For this review, take the finished solid that the model builds, in its own axes (mm). Face numbers are marked on the shaded views. A direction names the side the tool comes from. Give positions to 0.01 mm unless a question says otherwise; leave off trailing zeros. Loops run counter-clockwise (first coordinate to the right, second up) from the corner with the lowest first, then second, coordinate; pieces in that order, holes last.
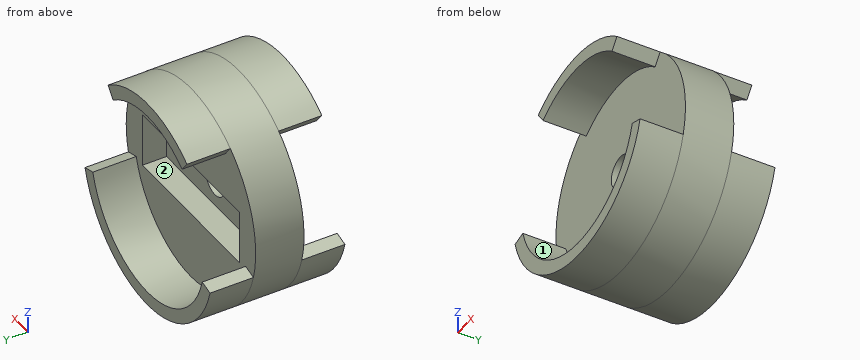
```python
from build123d import *

# Parameters (mm, degrees)
SKETCH1_R           = 25.4
SKETCH1_W           = 38.0365
SKETCH1_H           = 12.7508
BOSS_EXTRUDE1_DEPTH = 5.6642
SKETCH1_3_R         = 25.4
SKETCH1_3_W         = 38.0365
SKETCH1_3_H         = 12.7508
SKETCH1_3_R_2       = 3.71475
BOSS_EXTRUDE2_DEPTH = 5.715
BOSS_EXTRUDE3_DEPTH = 15.875


with BuildPart() as part:
    # Sketch1 → Boss-Extrude1 (new body)
    with BuildSketch(Plane(origin=(0, 0, 0), x_dir=(1, 0, 0), z_dir=(0, 1, 0))):
        Circle(SKETCH1_R)
        Rectangle(SKETCH1_W, SKETCH1_H, mode=Mode.SUBTRACT)
    extrude(amount=BOSS_EXTRUDE1_DEPTH)

    # Sketch1_3 → Boss-Extrude2 (add)
    with BuildSketch(Plane(origin=(0, 0, 0), x_dir=(1, 0, 0), z_dir=(0, 1, 0))):
        Circle(SKETCH1_3_R)
        Rectangle(SKETCH1_3_W, SKETCH1_3_H, mode=Mode.SUBTRACT)
        Rectangle(SKETCH1_3_W, SKETCH1_3_H)
        Circle(SKETCH1_3_R_2, mode=Mode.SUBTRACT)
    extrude(amount=-BOSS_EXTRUDE2_DEPTH)

    # Sketch2 → Boss-Extrude3 (add, symmetric)
    with BuildSketch(Plane(origin=(0, 0, 0), x_dir=(1, 0, 0), z_dir=(0, 1, 0))):
        with BuildLine():
            Line((21.467701, 5.752253), (24.534516, 6.574004))
            ThreePointArc((24.534516, 6.574004), (0, 25.4), (-24.534516, 6.574004))
            Line((-24.534516, 6.574004), (-21.467701, 5.752253))
            ThreePointArc((-21.467701, 5.752253), (0, 22.225), (21.467701, 5.752253))
        make_face()
        with BuildLine():
            Line((-13.529723, -17.632278), (-15.46254, -20.151175))
            ThreePointArc((-15.46254, -20.151175), (0, -25.4), (15.46254, -20.151175))
            Line((15.46254, -20.151175), (13.529723, -17.632278))
            ThreePointArc((13.529723, -17.632278), (0, -22.225), (-13.529723, -17.632278))
        make_face()
    extrude(amount=BOSS_EXTRUDE3_DEPTH, both=True)


solid = part.part
```
Item 1: For L1, parallel to X at y = -2, z = 0; L2, parallel to Y at x = 5, z = 12.5 (3 decimals); L3, parallel to Z at x = -21.5, y = -6.5, list the stretches that pass through material, from the lowest coordinate up.
Answer:
L1: x = -25.4 to -3.71, 3.71 to 25.4
L2: y = -5.715 to 5.664
L3: z = -13.52 to -5.76
Item 2: Take a section at A-A on z = 0. Give the boundary of the cut face in (x, y) (3 decimals), and give its area (3 significant figures).
Answer:
outline: (-25.4, -5.715) - (-3.715, -5.715) - (-3.715, 0) - (-19.018, 0) - (-19.018, 5.664) - (-25.4, 5.664) - close; (3.715, -5.715) - (25.4, -5.715) - (25.4, 5.664) - (19.018, 5.664) - (19.018, 0) - (3.715, 0) - close
area: 320 mm2
Item 3: Take a section at C-C on x = 0. Give the boundary of the cut face in (y, z) (3 decimals), and give its area (3 significant figures).
Answer:
outline: (-15.875, -25.4) - (15.875, -25.4) - (15.875, -22.225) - (5.664, -22.225) - (5.664, -6.375) - (0, -6.375) - (0, -3.715) - (-5.715, -3.715) - (-5.715, -22.225) - (-15.875, -22.225) - close; (-15.875, 22.225) - (-5.715, 22.225) - (-5.715, 3.715) - (0, 3.715) - (0, 6.375) - (5.664, 6.375) - (5.664, 22.225) - (15.875, 22.225) - (15.875, 25.4) - (-15.875, 25.4) - close
area: 593 mm2
Item 4: Clearance check with flat-ended pins moving along their axes: pin 1 Ø5 at (y, z) = (8.5, 18.5) entering from +X; pin 2 Ø4 at (y, z) = (-8.5, -19) entering from +X; pin 3 Ø10 at (y, z) = (2, -16) entering from +X. State where each tip first meets the part, or that it passes through.
Answer:
pin 1: stops at x = 15.46
pin 2: stops at x = 18.87
pin 3: stops at x = 22.89
Item 5: Take a section at B-B on y = 12. Give the boundary of the cut face in (x, z) (3 decimals).
Answer:
outline: (-24.535, -6.574) arc R25.4 ccw to (24.535, -6.574) - (21.468, -5.752) arc R22.225 cw to (-21.468, -5.752) - close; (-15.463, 20.151) - (-13.53, 17.632) arc R22.225 cw to (13.53, 17.632) - (15.463, 20.151) arc R25.4 ccw to start
Item 6: Tool access review of the marked faces 1 and 2: name each direction out of +Z, -Z, +X, -X, +Y, -Y from which nothing blocks a thin tool from reaching the whole face with its end or side.
Answer:
face 1: -Y
face 2: +Y
Item 7: Take a section at D-D on y = 4.5. Give the boundary of the cut face in (x, z), and give its area (3 significant figures).
Answer:
outline: circle Ø50.8 at (0, 0); hole (-19.02, -6.38) - (19.02, -6.38) - (19.02, 6.38) - (-19.02, 6.38) - close
area: 1,540 mm2
